Verification items for the finished model (mm, model axes). Face numbers are marked on the shaded views. A direction names the side the tool comes from. Give positions to 0.01 mm unless a question says otherwise; leave off trailing zeros. Loops run counter-clockwise (first coordinate to the right, second up) from the corner with the lowest first, then second, coordinate; pieces in that order, holes last. Notation, with made-up numbers: (11, 81.5) - (33, 81.5) arc R8 ccw to (33, 93.5) - close; hole circle Ø10 at (47, -27). An arc over 180 degrees is marked (long way). Use one line per item in the form item = value.
```python
from build123d import *

# Parameters (mm, degrees)
SKETCH1_W           = 70
SKETCH1_H           = 50
BOSS_EXTRUDE1_DEPTH = 6
CUT_EXTRUDE1_DEPTH  = 44.428101501
SKETCH3_W           = 15
SKETCH3_H           = 6
BOSS_EXTRUDE2_DEPTH = 25


with BuildPart() as part:
    # Sketch1 → Boss-Extrude1 (new body)
    with BuildSketch(Plane(origin=(0, 0, 0), x_dir=(1, 0, 0), z_dir=(0, 1, 0))):
        Rectangle(SKETCH1_W, SKETCH1_H)
    extrude(amount=BOSS_EXTRUDE1_DEPTH)

    # Sketch2 → Cut-Extrude1 (cut, through all)
    with BuildSketch(Plane.XZ):
        Polygon((-35, 12), (-20, 12), (-20, 37.174487296), (-39.665128523, 37.174487296), (-39.665128523, 12), align=None)
        Polygon((39.665128523, 12), (35, 12), (20, 12), (20, 37.174487296), (39.665128523, 37.174487296), align=None)
    extrude(amount=-CUT_EXTRUDE1_DEPTH, mode=Mode.SUBTRACT)

    # Sketch3 → Boss-Extrude2 (add)
    with BuildSketch(Plane.XZ):
        with Locations((-27.5, 9)):
            Rectangle(SKETCH3_W, SKETCH3_H)
        with Locations((27.5, 9)):
            Rectangle(SKETCH3_W, SKETCH3_H)
    extrude(amount=BOSS_EXTRUDE2_DEPTH)


solid = part.part
```
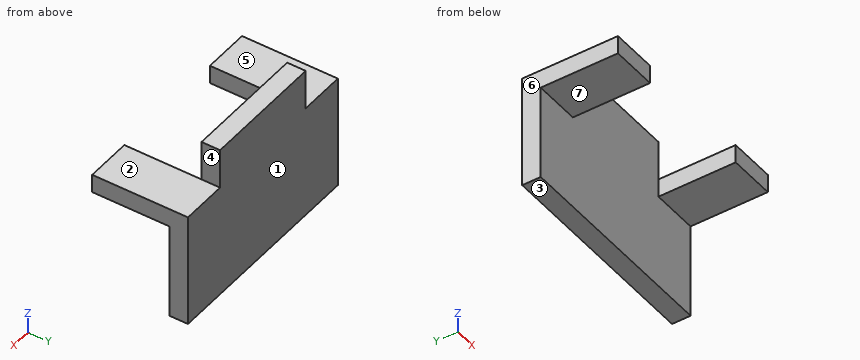
1. Section check A-A, the plane y = -18. Record the cut outline in (x, z).
Result set:
outline = (-35, 6) - (-20, 6) - (-20, 12) - (-35, 12) - close; (20, 6) - (35, 6) - (35, 12) - (20, 12) - close
2. Section check D-D, the plane x = -26. Record the cut outline in (y, z), then the cut area to 3 significant figures.
Result set:
outline = (-25, 6) - (0, 6) - (0, -25) - (6, -25) - (6, 12) - (-25, 12) - close
area = 372 mm²
3. Section check B-B, the plane y = 2. Record the cut outline in (x, z), then the cut area to 3 significant figures.
Result set:
outline = (-35, -25) - (35, -25) - (35, 12) - (20, 12) - (20, 25) - (-20, 25) - (-20, 12) - (-35, 12) - close
area = 3,110 mm²
4. Depth check by flat-ended pin: pin 1 Ø12 at (x, y) = (-27, -17) entering from -Z; pin 2 Ø1.8 at (y, z) = (4.5, 17) entering from +X; pin 3 Ø10 at (x, z) = (1, -15) entering from -Y. Enter the tip coordinate at first touch or a pass-through.
Result set:
pin_1 = 6
pin_2 = 20
pin_3 = 0
5. Scan lines: probe 1 along X at (y, z) = (-0.5, 10); probe 2 along Y at (x, z) = (15.5, -2); probe 3 along Z at (x, y) = (-26, -22.5). Record each from-to range of solid material in increasing order.
Result set:
probe_1 = -35 to -20, 20 to 35
probe_2 = 0 to 6
probe_3 = 6 to 12
6. Section check C-C, the plane z = 9.5. Record the cut outline in (x, y).
Result set:
outline = (-35, -25) - (-20, -25) - (-20, 0) - (20, 0) - (20, -25) - (35, -25) - (35, 6) - (-35, 6) - close
7. Draft check along Z on the marked faces 1, 2 and 3. Enter one of: released by +Z, released by -Z, zero draft, split by the parting line, or undercut.
Result set:
face_1 = zero draft
face_2 = released by +Z
face_3 = released by -Z
8. Tool access check on the marked faces 4, 5, 6 and 7. Record the directions out of +Z, -Z, +X, -X, +Y, -Y that give a thin tool (end or side, any length) a straight path to the whole face; none if there is none.
Result set:
face_4 = +Z, +X, +Y, -Y
face_5 = +Z, -X, +Y, -Y
face_6 = +Z, -Z, -X, +Y, -Y
face_7 = -Z, +X, -X, -Y
